For this review, take the finished solid that the model builds, in its own axes (mm). Round coordinates to 2 decimals unless told otherwise and drop trailing zeros. Loops run counter-clockwise (first coordinate to the right, second up) from the corner with the lowest first, then second, coordinate; pieces in that order, holes last. Notation, with made-up numbers: (39, -36.5) -> (90, -36.5) arc R23 ccw to (90, -7.5) -> close; hole circle Ø10 at (-25, 32). An arc over 180 degrees is marked (long way). Write each question's results on one line, items separated by ' | '.
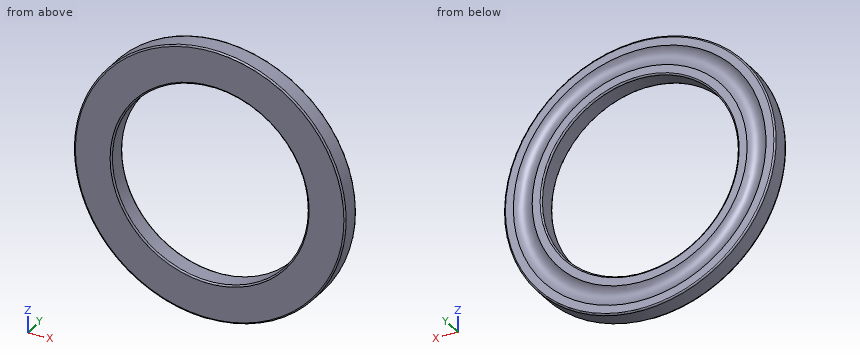
```python
from build123d import *

# Parameters (mm, degrees)
FILLET1_R = 0.5


with BuildPart() as part:
    # Sketch1 → Revolve1 (revolve)
    with BuildSketch(Plane.XY):
        with BuildLine():
            Line((32.5, 0), (45, 0))
            Line((45, 0), (45, 6.5))
            Line((45, 6.5), (41.872498999, 6.5))
            ThreePointArc((41.872498999, 6.5), (38.75, 5), (35.627501001, 6.5))
            Line((35.627501001, 6.5), (32.5, 6.5))
            Line((32.5, 6.5), (32.5, 0))
        make_face()
    revolve(axis=Axis((0, 0, 0), (0, 1, 0)))

    # Fillet1
    fillet1_edges = [part.edges().sort_by_distance(p)[0] for p in [
        (-32.5, 6.5, 0),
        (-45, 6.5, 0),
        (-45, 0, 0),
        (-32.5, 0, 0),
    ]]
    fillet(fillet1_edges, radius=FILLET1_R)


solid = part.part
```
1. To check wall thickness, follow probe 1 along Z at (x, y) = (7, 6.25); probe 2 along Z at (x, y) = (0, 3.55). State the ranges of each line that lie inside material, in increasing order.
Values found:
probe 1: z = -44.38 to -41.06, -35.16 to -31.81, 31.81 to 35.16, 41.06 to 44.38 | probe 2: z = -45 to -32.5, 32.5 to 45
2. Consider section A-A (z = 0). State the section outline as (x, y) points.
Values found:
outline: (-45, 0.5) arc R0.5 ccw to (-44.5, 0) -> (-33, 0) arc R0.5 ccw to (-32.5, 0.5) -> (-32.5, 6) arc R0.5 ccw to (-33, 6.5) -> (-35.63, 6.5) arc R4 cw to (-41.87, 6.5) -> (-44.5, 6.5) arc R0.5 ccw to (-45, 6) -> close; (32.5, 0.5) arc R0.5 ccw to (33, 0) -> (44.5, 0) arc R0.5 ccw to (45, 0.5) -> (45, 6) arc R0.5 ccw to (44.5, 6.5) -> (41.87, 6.5) arc R4 cw to (35.63, 6.5) -> (33, 6.5) arc R0.5 ccw to (32.5, 6) -> close
3. Consider section C-C (y = 2.5). State the section outline as (x, z) points.
Values found:
outline: circle Ø90 at (0, 0); hole circle Ø65 at (0, 0)
4. Consider section B-B (x = 0). State the section outline as (y, z) points.
Values found:
outline: (0, -44.5) arc R0.5 ccw to (0.5, -45) -> (6, -45) arc R0.5 ccw to (6.5, -44.5) -> (6.5, -41.87) arc R4 cw to (6.5, -35.63) -> (6.5, -33) arc R0.5 ccw to (6, -32.5) -> (0.5, -32.5) arc R0.5 ccw to (0, -33) -> close; (0, 33) arc R0.5 ccw to (0.5, 32.5) -> (6, 32.5) arc R0.5 ccw to (6.5, 33) -> (6.5, 35.63) arc R4 cw to (6.5, 41.87) -> (6.5, 44.5) arc R0.5 ccw to (6, 45) -> (0.5, 45) arc R0.5 ccw to (0, 44.5) -> close
5. For pin 1 (1.5 mm diameter, centred on x = -15.5, y = 4.5, fed in from +Z); pin 2 (2 mm diameter, centred on y = 4, z = 16.5, fed in from -X); pin 3 (5 mm diameter, centred on x = -33.5, z = -23, fed in from -Y); pin 4 (1 mm diameter, centred on x = 31, y = 5, fed in from -Z), all flat-tipped, find the tip position at first contact; note any pin that passes through.
Values found:
pin 1: stops at z = 42.51 | pin 2: stops at x = -42.25 | pin 3: stops at y = 0 | pin 4: stops at z = -33.09
